Build history of the part. All positions in model axes, mm. Coordinates: 2 decimals unless noted, no trailing zeros. Order: outer loops, then holes, each group sorted by start corner. A loop starts at its lowest first (then second) coordinate and runs counter-clockwise, first axis right, second up. Notation, with made-up numbers: M -25.5,82 L 8.5,82 A30 ccw 8.5,118 Z; hole C 44,-35 d3. An arc over 180 degrees is marked long. Write item = value, one per line. Start each with the question number.
Q1. Band-saw the part on A-A on x = -40. Write the cut outline in (y, z).
Q2. Drill centre lines: probe 1 along Z at (x, y) = (-46, 5); probe 2 along Y at (x, z) = (-45, 22). Where is each one in solid material? Low to high.
Q3. Pin check, flat tips, straight feed: P1, Ø2, axis at y = 5, z = 22, coming from the +X side; P2, Ø5.5, axis at y = 5, z = 0, coming from the +X side; P3, Ø3, axis at y = 5, z = -22, coming from the -X side; P4, Ø2, axis at y = 5, z = -22, coming from the -X side. Stop position of each tip, or through.
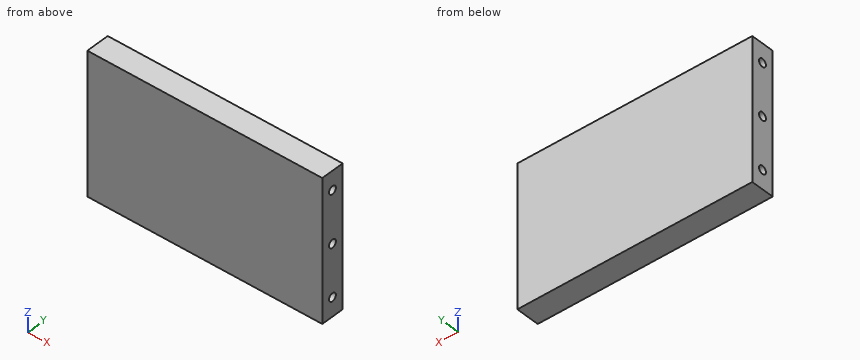
```python
from build123d import *

# Parameters (mm, degrees)
SKETCH1_W                      = 100
SKETCH1_H                      = 60
BOSS_EXTRUDE1_DEPTH            = 10
CBORE_FOR_M3_SHCS1_D           = 3.4
CBORE_FOR_M3_SHCS1_DEPTH       = 23
CBORE_FOR_M3_SHCS1_CBORE_D     = 6.5
CBORE_FOR_M3_SHCS1_CBORE_DEPTH = 3
CBORE_FOR_M3_SHCS1_TIP         = 1.021463052
CBORE_FOR_M3_SHCS2_D           = 3.4
CBORE_FOR_M3_SHCS2_DEPTH       = 23
CBORE_FOR_M3_SHCS2_CBORE_D     = 6.5
CBORE_FOR_M3_SHCS2_CBORE_DEPTH = 3
CBORE_FOR_M3_SHCS2_TIP         = 1.021463052


with BuildPart() as part:
    # Sketch1 → Boss-Extrude1 (new body)
    with BuildSketch(Plane(origin=(0, 0, 0), x_dir=(1, 0, 0), z_dir=(0, 1, 0))):
        Rectangle(SKETCH1_W, SKETCH1_H)
    extrude(amount=BOSS_EXTRUDE1_DEPTH)

    # CBORE for M3 SHCS1
    with Locations(Plane(origin=(60, -888.012147263, -1303.282701689), x_dir=(0, 0, -1), z_dir=(1, 0, 0))):
        with Locations((-1281.282701689, 893.012147263), (-1325.282701689, 893.012147263), (-1303.282701689, 893.012147263)):
            CounterBoreHole(CBORE_FOR_M3_SHCS1_D / 2, CBORE_FOR_M3_SHCS1_CBORE_D / 2, CBORE_FOR_M3_SHCS1_CBORE_DEPTH, depth=CBORE_FOR_M3_SHCS1_DEPTH)
            with Locations((0, 0, -(CBORE_FOR_M3_SHCS1_DEPTH + CBORE_FOR_M3_SHCS1_TIP / 2))):  # 118° drill point
                Cone(0, CBORE_FOR_M3_SHCS1_D / 2, CBORE_FOR_M3_SHCS1_TIP, mode=Mode.SUBTRACT)

    # CBORE for M3 SHCS2
    with Locations(Plane(origin=(-60, -888.012147263, -1303.282701689), x_dir=(0, 0, 1), z_dir=(-1, 0, 0))):
        with Locations((1281.282701689, 893.012147263), (1325.282701689, 893.012147263), (1303.282701689, 893.012147263)):
            CounterBoreHole(CBORE_FOR_M3_SHCS2_D / 2, CBORE_FOR_M3_SHCS2_CBORE_D / 2, CBORE_FOR_M3_SHCS2_CBORE_DEPTH, depth=CBORE_FOR_M3_SHCS2_DEPTH)
            with Locations((0, 0, -(CBORE_FOR_M3_SHCS2_DEPTH + CBORE_FOR_M3_SHCS2_TIP / 2))):  # 118° drill point
                Cone(0, CBORE_FOR_M3_SHCS2_D / 2, CBORE_FOR_M3_SHCS2_TIP, mode=Mode.SUBTRACT)


solid = part.part
```
Recorded:
q1.outline = M 0,-30 L 10,-30 L 10,30 L 0,30 Z; hole C 5,-22 d3.4; hole C 5,0 d3.4; hole C 5,22 d3.4
q2.probe_1 = -30 to -23.7, -20.3 to -1.7, 1.7 to 20.3, 23.7 to 30
q2.probe_2 = 0 to 3.3, 6.7 to 10
q3.P1 = 36.58
q3.P2 = 50
q3.P3 = -36.88
q3.P4 = -36.58
